from build123d import *

# Parameters (mm, degrees)
F2_SIZE  = 0.508
F3_SIZE  = 0.508
F5_DEPTH = 9.525


with BuildPart() as f1:
    # F0 (on Top) → F1 (revolve)
    with BuildSketch(Plane.XY):
        Polygon((-9.525, -1.905), (0, -1.905), (0, 1.905), (-12.7, 1.905), (-19.05, 1.905), (-19.05, -1.905), align=None)
        with BuildLine():
            Line((0, -22.479), (0, -1.905))
            Line((0, -1.905), (-9.525, -1.905))
            ThreePointArc((-9.525, -1.905), (-8.55091, -2.87909), (-9.525, -3.85318))
            Line((-9.525, -3.85318), (-9.525, -22.479))
            Line((-9.525, -22.479), (0, -22.479))
        make_face()
        with BuildLine():
            Line((-12.7, 1.905), (0, 1.905))
            Line((0, 1.905), (0, 36.83))
            Line((0, 36.83), (-12.7, 36.83))
            Line((-12.7, 36.83), (-12.7, 3.85318))
            ThreePointArc((-12.7, 3.85318), (-11.72591, 2.87909), (-12.7, 1.905))
        make_face()
    revolve(axis=Axis((0, 7.1755, 0), (0, -1, 0)))

    # F2
    f2_edges = [f1.edges().sort_by_distance(p)[0] for p in [
        (12.7, 36.83, 0),
    ]]
    chamfer(f2_edges, length=F2_SIZE)

    # F3
    f3_edges = [f1.edges().sort_by_distance(p)[0] for p in [
        (19.05, -1.905, 0),
    ]]
    chamfer(f3_edges, length=F3_SIZE)

    # F4 (on face) → F5 (cut)
    with BuildSketch(Plane(origin=(0, 36.83, 0), x_dir=(-1, 0, 0), z_dir=(0, 1, 0))):
        with BuildLine():
            Line((-7.6104690394, 9.525), (7.6104690394, 9.525))
            ThreePointArc((7.6104690394, 9.525), (0, 12.192), (-7.6104690394, 9.525))
        make_face()
        with BuildLine():
            Line((7.6104690394, 9.525), (12.7, 9.525))
            Line((12.7, 9.525), (12.7, 12.7))
            Line((12.7, 12.7), (-12.7, 12.7))
            Line((-12.7, 12.7), (-12.7, 9.525))
            Line((-12.7, 9.525), (-7.6104690394, 9.525))
            ThreePointArc((-7.6104690394, 9.525), (0, 12.192), (7.6104690394, 9.525))
        make_face()
        with BuildLine():
            Line((-12.7, -12.7), (12.7, -12.7))
            Line((12.7, -12.7), (12.7, -9.525))
            Line((12.7, -9.525), (7.6104690394, -9.525))
            ThreePointArc((7.6104690394, -9.525), (0, -12.192), (-7.6104690394, -9.525))
            Line((-7.6104690394, -9.525), (-12.7, -9.525))
            Line((-12.7, -9.525), (-12.7, -12.7))
        make_face()
        with BuildLine():
            ThreePointArc((-7.6104690394, -9.525), (0, -12.192), (7.6104690394, -9.525))
            Line((7.6104690394, -9.525), (-7.6104690394, -9.525))
        make_face()
    extrude(amount=-F5_DEPTH, mode=Mode.SUBTRACT)


solid = f1.part
The listing builds one solid part. Answer for the finished solid, in the listing's coordinates (mm). A direction names the side the tool comes from. Give positions to 0.01 mm unless a question says otherwise; leave off trailing zeros. Write each loop counter-clockwise with the first axis right and the second up, starting at its lowest first coordinate (ties: lowest second). Pieces come first, ordered by that corner, then holes. Notation, with made-up numbers: (-4.75, -9) - (34.25, -9) arc R12 ccw to (34.25, 4) - close; hole circle Ø1 at (23, 59). An arc over 180 degrees is marked (long way). One line per question, with ' | ' between items. Start each with the question number.
1. Section A-A, the plane z = 0 is taken. Determine the outline of the cut face in (x, y) (3 decimals), then the cut area to 3 significant figures.
2. For faces 1 (the face through (0, 32, -9.525)), 2 (the face through (12.4, 1.905, 4)), 3 (the face through (9, -1.905, -4)), determine the directions among +Z, -Z, +X, -X, +Y, -Y from which every point of the face is accessible in a straight line to the end or side of a thin tool.
3. Straight lines are drawn through the part: line 1 (Y direction, x = 7, z = 13.5) (3 decimals); line 2 (Y direction, x = 0, z = 11.5) (3 decimals); line 3 (Y direction, x = -3.5, z = 12) (3 decimals). For each, find the intervals that lie inside material, in ascending order.
4. Section C-C, the plane y = 31 is taken. Determine the outline of the cut face in (x, z) (3 decimals), then the cut area to 3 significant figures.
5. Section D-D, the plane y = -12 is taken. Determine the outline of the cut face in (x, z) (3 decimals), then the cut area to 3 significant figures.
6. Given P1, Ø7.5, axis at x = 0, y = 32, coming from the +Z side (3 decimals); P2, Ø2, axis at x = -7, y = 4.5, coming from the -Z side; P3, Ø5, axis at y = 28, z = 11, coming from the +X side, each flat-ended and moving along its own axis, determine where each tip first touches the part or whether it passes through.
7. Section B-B, the plane x = 0 is taken. Determine the outline of the cut face in (y, z) (3 decimals).
Result:
1) outline: (-19.05, -1.397) - (-18.542, -1.905) - (-9.525, -1.905) arc R0.974 cw to (-9.525, -3.853) - (-9.525, -22.479) - (9.525, -22.479) - (9.525, -3.853) arc R0.974 cw to (9.525, -1.905) - (18.542, -1.905) - (19.05, -1.397) - (19.05, 1.905) - (12.7, 1.905) arc R0.974 cw to (12.7, 3.853) - (12.7, 36.322) - (12.192, 36.83) - (-12.192, 36.83) - (-12.7, 36.322) - (-12.7, 3.853) arc R0.974 cw to (-12.7, 1.905) - (-19.05, 1.905) - close | area: 1,420 mm2
2) face 1: -Z, +X, -X, +Y | face 2: +Y | face 3: -Y
3) line 1: y = -1.905 to 1.905 | line 2: y = -1.905 to 27.305 | line 3: y = -1.905 to 1.926, 3.832 to 27.305
4) outline: (-8.4, -9.525) - (8.4, -9.525) arc R12.7 ccw to (8.4, 9.525) - (-8.4, 9.525) arc R12.7 ccw to start | area: 434 mm2
5) outline: circle Ø19.05 at (0, 0) | area: 285 mm2
6) P1: stops at z = 9.525 | P2: stops at z = -11.19 | P3: stops at x = 9.44
7) outline: (-22.479, -9.525) - (-3.853, -9.525) arc R0.974 cw to (-1.905, -9.525) - (-1.905, -18.542) - (-1.397, -19.05) - (1.905, -19.05) - (1.905, -12.7) arc R0.974 cw to (3.853, -12.7) - (27.305, -12.7) - (27.305, -9.525) - (36.83, -9.525) - (36.83, 9.525) - (27.305, 9.525) - (27.305, 12.7) - (3.853, 12.7) arc R0.974 cw to (1.905, 12.7) - (1.905, 19.05) - (-1.397, 19.05) - (-1.905, 18.542) - (-1.905, 9.525) arc R0.974 cw to (-3.853, 9.525) - (-22.479, 9.525) - close
